The listing builds one solid part. Answer for the finished solid, in the listing's coordinates (mm). A direction names the side the tool comes from. Coordinates: 2 decimals unless noted, no trailing zeros. Order: outer loops, then holes, each group sorted by start corner. A loop starts at its lowest first (then second) coordinate and runs counter-clockwise, first axis right, second up.
```python
from build123d import *

# Parameters (mm, degrees)
SKETCH1_R           = 4.05
SKETCH1_R_2         = 1.7
SKETCH1_R_3         = 8.05
BOSS_EXTRUDE1_DEPTH = 5


with BuildPart() as part:
    # Sketch1 → Boss-Extrude1 (new body)
    with BuildSketch(Plane.XY):
        Polygon((32.079048784, 30), (-37.5, 30), (-37.5, -35), (40.987000641, -35), (60.75120914, -15.235791501), (60.75120914, 5.94120082), align=None)
        with Locations((16, 20)):
            Circle(SKETCH1_R, mode=Mode.SUBTRACT)
        with Locations((50, 0)):
            Circle(SKETCH1_R, mode=Mode.SUBTRACT)
        with Locations((-18.5, -15)):
            Circle(SKETCH1_R, mode=Mode.SUBTRACT)
        with Locations((30.987000641, -30)):
            Circle(SKETCH1_R_2, mode=Mode.SUBTRACT)
        Circle(SKETCH1_R_3, mode=Mode.SUBTRACT)
        with BuildLine():
            Line((53.231228952, -6.031636678), (54.952673272, -7.751314072))
            ThreePointArc((54.952673272, -7.751314072), (54.953907747, -10.155476811), (52.549745008, -10.156711286))
            Line((52.549745008, -10.156711286), (50.828300688, -8.437033892))
            ThreePointArc((50.828300688, -8.437033892), (50.827066213, -6.032871153), (53.231228952, -6.031636678))
        make_face(mode=Mode.SUBTRACT)
        with BuildLine():
            ThreePointArc((29.199069372, 15.505889539), (30.987000641, 15.541), (32.774931911, 15.505889539))
            ThreePointArc((32.774931911, 15.505889539), (34.406879586, 13.740458491), (32.641448537, 12.108510816))
            ThreePointArc((32.641448537, 12.108510816), (30.987000641, 12.141), (29.332552745, 12.108510816))
            ThreePointArc((29.332552745, 12.108510816), (27.567121697, 13.740458491), (29.199069372, 15.505889539))
        make_face(mode=Mode.SUBTRACT)
        with BuildLine():
            ThreePointArc((29.529218906, 3.388691089), (30.987000641, 3.4205), (32.444782377, 3.388691089))
            ThreePointArc((32.444782377, 3.388691089), (43.43221397, -8.601986414), (31.441536467, -19.589418007))
            ThreePointArc((31.441536467, -19.589418007), (30.987000641, -19.5795), (30.532464815, -19.589418007))
            ThreePointArc((30.532464815, -19.589418007), (18.541787312, -8.601986414), (29.529218906, 3.388691089))
        make_face(mode=Mode.SUBTRACT)
    extrude(amount=BOSS_EXTRUDE1_DEPTH)


solid = part.part
```
(1) Each of these flat-tipped pins is pushed along its axis until it touches: pin 1 Ø5 at (x, y) = (16, 20) entering from +Z; pin 2 Ø2 at (y, z) = (-20.5, 0.5) entering from +X. Where does it stop, or does it pass through?
(2) Consider line 1 (Y direction, x = 0, z = 2.8); line 2 (Y direction, x = -18.5, z = 3.05); line 3 (X direction, y = -4.5, z = 1.9). Determine where each line is inside the solid, lowest interval first.
(3) Find section B-B (y = 20). Write down the section's boundary in (x, z), and give its area (3 significant figures).
(4) Find section C-C (z = 3.1). Give the number of separate pieces and of enclosed holes in the cut face, and give its area (3 significant figures).
(5) The mould has two halves that part along Y. Classify faces 3 (the face through (30.97, 3.42, 2.46)), 4 (the face through (-37.5, -2, 2)), 5 (the face through (-2, 30, 2)): released by +Y, released by -Y, zero draft, split by the parting line, or undercut.
(6) Find section A-A (x = 0). Write down the section's boundary in (y, z), and give its area (4 significant figures).
(7) For faces 1 (the face through (31.01, 12.14, 2.46)), 2 (the face through (60.751, -5, 2)), determine the directions among +Z, -Z, +X, -X, +Y, -Y from which every point of the face is accessible in a straight line to the end or side of a thin tool.
Findings below:
1. pin 1: passes through
1. pin 2: stops at x = 56.49
2. line 1: y = -35 to -8.05, 8.05 to 30
2. line 2: y = -35 to -19.05, -10.95 to 30
2. line 3: x = -37.5 to -6.67, 6.67 to 19.11, 42.87 to 60.75
3. outline: (-37.5, 0) - (11.95, 0) - (11.95, 5) - (-37.5, 5) - close; (20.05, 0) - (44, 0) - (44, 5) - (20.05, 5) - close
3. area: 367 mm2
4. separate pieces: 1
4. enclosed holes: 8
4. area: 4,980 mm2
5. face 3: undercut
5. face 4: zero draft
5. face 5: released by +Y
6. outline: (-35, 0) - (-8.05, 0) - (-8.05, 5) - (-35, 5) - close; (8.05, 0) - (30, 0) - (30, 5) - (8.05, 5) - close
6. area: 244.5 mm2
7. face 1: +Z, -Z
7. face 2: +Z, -Z, +X, +Y, -Y
